Check sheet for the modelled part. Datum: model origin and axes. Units: mm. Round coordinates to 2 decimals unless told otherwise and drop trailing zeros. Write each loop counter-clockwise with the first axis right and the second up, starting at its lowest first coordinate (ties: lowest second). Pieces come first, ordered by that corner, then holes.
Item 1: Cross-section at A-A on x = 0. Enter the section's corners in (y, z).
Item 2: Material ranges on line 1 (Y direction, x = 0, z = 10); line 2 (X direction, y = -1, z = 13.5); line 3 (Z direction, x = -2, y = -10.25), recorded low to high.
Item 3: Cross-section at C-C on z = 8. Enter the section's corners in (x, y), plus the area to 3 significant figures.
Item 4: Release check for a two-part mould opening along Y. For faces 1 (the flat face through (0, -7, 0)), 2 (the cylindrical face through (-0.74, -3.32, 9.62)), 3 (the cylindrical face through (11.923, 3.755, 9.427)) record: +Y half, -Y half, draft (parallel to the pull), parting line (faces both ways), or undercut.
Item 5: Go/stop test with flat-tipped pins: pin 1 Ø4 at (x, y) = (0, 0) entering from -Z; pin 2 Ø2 at (y, z) = (2.5, 5) entering from -X; pin 3 Ø8 at (y, z) = (9, 15.5) entering from -X; pin 4 Ø10 at (x, y) = (9.5, -8) entering from -Z. Record where each tip stops, or that it passes through.
from build123d import *

# Parameters (mm, degrees)
F0_R     = 12.5
F1_DEPTH = 19.05
F2_R     = 3.4
F3_DEPTH = 25.4
F4_SIZE  = 2.54


with BuildPart() as f1:
    # F0 (on Top) → F1 (new body)
    with BuildSketch(Plane.XY):
        Circle(F0_R)
    extrude(amount=F1_DEPTH)

    # F2 (on face) → F3 (cut)
    with BuildSketch(Plane.XY.offset(19.05)):
        Circle(F2_R)
    extrude(amount=-F3_DEPTH, mode=Mode.SUBTRACT)

    # F4
    f4_edges = [f1.edges().sort_by_distance(p)[0] for p in [
        (-3.4, 0, 19.05),
        (-3.4, 0, 0),
        (-12.5, 0, 0),
        (-12.5, 0, 19.05),
    ]]
    chamfer(f4_edges, length=F4_SIZE)


solid = f1.part
Response values:
1. outline: (-12.5, 2.54) - (-9.96, 0) - (-5.94, 0) - (-3.4, 2.54) - (-3.4, 16.51) - (-5.94, 19.05) - (-9.96, 19.05) - (-12.5, 16.51) - close; (3.4, 2.54) - (5.94, 0) - (9.96, 0) - (12.5, 2.54) - (12.5, 16.51) - (9.96, 19.05) - (5.94, 19.05) - (3.4, 16.51) - close
2. line 1: y = -12.5 to -3.4, 3.4 to 12.5
2. line 2: x = -12.46 to -3.25, 3.25 to 12.46
2. line 3: z = 0.48 to 18.57
3. outline: circle Ø25 at (0, 0); hole circle Ø6.8 at (0, 0)
3. area: 455 mm2
4. face 1: draft
4. face 2: undercut
4. face 3: parting line
5. pin 1: passes through
5. pin 2: stops at x = -12.41
5. pin 3: stops at x = -11.46
5. pin 4: stops at z = 0
